Input: part model. Units: mm. Frame: model coordinates. A direction names the side the tool comes from. Give positions to 0.01 mm unless a question says otherwise; leave off trailing zeros. Order: outer loops, then holes, each group sorted by start corner. A loop starts at its lowest first (then second) coordinate and runs counter-clockwise, first axis right, second up. Notation, with made-up numbers: (56.5, 39) - (97.5, 39) arc R10 ccw to (97.5, 51) - close; hole circle Ø11 at (69, 89). An arc over 180 degrees is marked (long way). Answer in a Markdown table with one row per item. Add a question column.
1. Section query A-A on z = -2.5. Return loops of the section in (x, y).
2. Section query C-C on x = 0. Return loops of the section in (y, z) (1 decimal), and give its area (3 significant figures).
3. Mould query, pull axis X, two halves, no side actions, for faces 1 (the face through (-9, -2, -22)), 2 (the face through (-6.137, 2.766, -0.815)), 3 (the face through (-1, 7, -25.86)). Classes: released by +X, released by -X, zero draft, split by the parting line, or undercut.
4. Section query B-B on y = 0. Return loops of the section in (x, z) (1 decimal).
5. Section query D-D on z = 20. Return loops of the section in (x, y).
6. Ray query, line 1 (X direction, y = -2.25, z = 19.5); line 2 (Y direction, x = 1.5, z = -17); line 3 (Y direction, x = 0.5, z = -21.5). Return the intervals inside material, ascending. Write a range as [from, to].
7. Access query for faces 4 (the face through (1, -7, 24.94)), 5 (the face through (5.464, 3.932, -0.815)). Directions: +Z, -Z, +X, -X, +Y, -Y. A direction counts if a zero-diameter tool reaches every point of the face in a straight line with its end or side. Return the directions, or none.
8. Contact query for flat-ended pins moving along their axis: pin 1 (6 mm diameter, centred on y = -7.5, z = -6, fed in from -X); pin 2 (2 mm diameter, centred on x = -3, y = 4, fed in from -Z); pin 3 (5 mm diameter, centred on x = -3.5, z = 6.5, fed in from -Y); pin 4 (1.5 mm diameter, centred on y = -0.5, z = 15.5, fed in from -X). Output: stop coordinate, or through.
```python
from build123d import *

# Parameters (mm, degrees)
F3_DEPTH      = 38.1
F3_DEPTH_BACK = 38.1


with BuildPart() as f2:
    # F1 (on Right) → F2 (revolve)
    with BuildSketch(Plane.YZ):
        Polygon((8.255, 24.9404996053), (6.731, 24.9404996053), (6.731, -25.8595003947), (8.255, -25.8595003947), (11.43, -13.1595003947), (11.43, 12.2404996053), align=None)
    revolve(axis=Axis((0, 0, -0.0453809016), (0, 0, -1)))

    # F0 (on Top) → F3 (cut, two sides)
    with BuildSketch(Plane.XY) as f3_sk:
        Polygon((7.7267937867, 0.8397256168), (3.136173177, 7.1114625174), (-4.5906206097, 6.2717369007), (-7.7267937867, -0.8397256168), (-3.136173177, -7.1114625174), (4.5906206097, -6.2717369007), align=None)
    extrude(amount=-F3_DEPTH, mode=Mode.SUBTRACT)
    extrude(f3_sk.sketch, amount=F3_DEPTH_BACK, mode=Mode.SUBTRACT)


solid = f2.part
```
Answer:
| question | item | result |
|---|---|---|
| 1 | outline | circle Ø22.86 at (0, 0); hole (-7.73, -0.84) - (-3.14, -7.11) - (4.59, -6.27) - (7.73, 0.84) - (3.14, 7.11) - (-4.59, 6.27) - close |
| 2 | outline | (-11.4, -13.2) - (-8.3, -25.9) - (-6.8, -25.9) - (-6.8, 24.9) - (-8.3, 24.9) - (-11.4, 12.2) - close; (6.8, -25.9) - (8.3, -25.9) - (11.4, -13.2) - (11.4, 12.2) - (8.3, 24.9) - (6.8, 24.9) - close |
| 2 | area | 393 mm² |
| 3 | face 1 | split by the parting line |
| 3 | face 2 | undercut |
| 3 | face 3 | zero draft |
| 4 | outline | (-11.4, -13.2) - (-8.3, -25.9) - (-7.4, -25.9) - (-7.4, 24.9) - (-8.3, 24.9) - (-11.4, 12.2) - close; (7.4, -25.9) - (8.3, -25.9) - (11.4, -13.2) - (11.4, 12.2) - (8.3, 24.9) - (7.4, 24.9) - close |
| 5 | outline | circle Ø18.98 at (0, 0); hole (-7.73, -0.84) - (-3.14, -7.11) - (4.59, -6.27) - (7.73, 0.84) - (3.14, 7.11) - (-4.59, 6.27) - close |
| 6 | line 1 | x = [-9.35, -6.69], [6.36, 9.35] |
| 6 | line 2 | y = [-10.36, -6.61], [6.93, 10.36] |
| 6 | line 3 | y = [-9.33, -6.72], [6.82, 9.33] |
| 7 | face 4 | +Z, +X, -X, +Y, -Y |
| 7 | face 5 | +Z, -Z |
| 8 | pin 1 | stops at x = -10.51 |
| 8 | pin 2 | passes through |
| 8 | pin 3 | stops at y = -11.39 |
| 8 | pin 4 | stops at x = -10.79 |
